from build123d import *

# Parameters (mm, degrees)
PAD_DEPTH     = 5
SKETCH001_R   = 7.925
SKETCH001_R_2 = 32.55
SKETCH001_R_3 = 25.8
SKETCH001_R_4 = 11.5
PAD001_DEPTH  = 2


with BuildPart() as part:
    # Sketch → Pad (new body)
    with BuildSketch(Plane.XY):
        with BuildLine():
            ThreePointArc((0, 8.25), (2.416369, 2.416369), (8.25, 0))
            Line((80.65, 0), (8.25, 0))
            ThreePointArc((80.65, 0), (86.483631, 2.416369), (88.9, 8.25))
            Line((88.9, 88.75), (88.9, 8.25))
            ThreePointArc((88.9, 88.75), (86.483631, 94.583631), (80.65, 97))
            Line((8.25, 97), (80.65, 97))
            ThreePointArc((8.25, 97), (2.416369, 94.583631), (0, 88.75))
            Line((0, 8.25), (0, 88.75))
        make_face()
    extrude(amount=PAD_DEPTH)

    # Sketch001 (on Face10 of Pad) → Pad001 (join)
    with BuildSketch(Plane.XY.offset(5)):
        with Locations((16.275, 80.075)):
            Circle(SKETCH001_R)
        with Locations((44.45, 44.45)):
            Circle(SKETCH001_R_2)
        with Locations((44.45, 44.45)):
            Circle(SKETCH001_R_3, mode=Mode.SUBTRACT)
        with Locations((44.45, 44.45)):
            Circle(SKETCH001_R_4)
    extrude(amount=PAD001_DEPTH)


solid = part.part
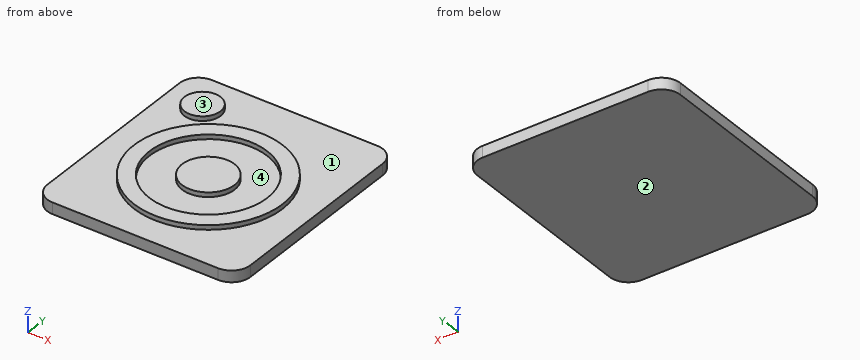
Input: part model. Units: mm. Frame: model coordinates. Face numbers are marked on the shaded views. A direction names the side the tool comes from. Round coordinates to 2 decimals unless told otherwise and drop trailing zeros. Write each loop counter-clockwise with the first axis right and the second up, starting at its lowest first coordinate (ties: lowest second). Pieces come first, ordered by that corner, then holes.
1) Cut plane D-D (y = 16). Return the cut outline in (x, z), then the cut area to 3 significant figures.
2) Ray query, L1, parallel to Y at x = 44.45, z = 5.6; L2, parallel to Z at x = 19, y = 91.5; L3, parallel to Y at x = 53, z = 6.5. Return the intervals inside material, ascending.
3) Contact query for flat-ended pins moving along their axis: P1, Ø6, axis at x = 78, y = 24, coming from the +Z side; P2, Ø5, axis at x = 23, y = 23, coming from the -Z side. Output: stop coordinate, or through.
4) Draft query along Y for the marked faces 3 and 4. Return one class per face: pulls with the +Y half, pulls with the -Y half, needs draft (parallel to the pull), parting line crosses it, or undercut.
5) Reachability of the marked faces 1 and 2 from +Z, -Z, +X, -X, +Y, -Y: full face, straight path, thin tool, end or side. Return the list, or none.
6) Cut plane C-C (x = 44.45). Return the cut outline in (y, z), then the cut area to 3 significant figures.
7) Cut plane A-A (y = 44.45). Return the cut outline in (x, z).
8) Cut plane B-B (x = 29.5). Return the cut outline in (y, z).
Geometry says:
1. outline: (0, 0) - (88.9, 0) - (88.9, 5) - (60.26, 5) - (60.26, 7) - (28.64, 7) - (28.64, 5) - (0, 5) - close
1. area: 508 mm2
2. L1: y = 11.9 to 18.65, 32.95 to 55.95, 70.25 to 77
2. L2: z = 0 to 5
2. L3: y = 13.04 to 20.11, 36.76 to 52.14, 68.79 to 75.86
3. P1: stops at z = 5
3. P2: stops at z = 0
4. face 3: needs draft
4. face 4: undercut
5. face 1: +Z
5. face 2: -Z, +X, -X, +Y, -Y
6. outline: (0, 0) - (97, 0) - (97, 5) - (77, 5) - (77, 7) - (70.25, 7) - (70.25, 5) - (55.95, 5) - (55.95, 7) - (32.95, 7) - (32.95, 5) - (18.65, 5) - (18.65, 7) - (11.9, 7) - (11.9, 5) - (0, 5) - close
6. area: 558 mm2
7. outline: (0, 0) - (88.9, 0) - (88.9, 5) - (77, 5) - (77, 7) - (70.25, 7) - (70.25, 5) - (55.95, 5) - (55.95, 7) - (32.95, 7) - (32.95, 5) - (18.65, 5) - (18.65, 7) - (11.9, 7) - (11.9, 5) - (0, 5) - close
8. outline: (0, 0) - (97, 0) - (97, 5) - (73.36, 5) - (73.36, 7) - (65.48, 7) - (65.48, 5) - (23.42, 5) - (23.42, 7) - (15.54, 7) - (15.54, 5) - (0, 5) - close
